Design review of the part built by this model. Coordinates are the model's own, in mm. A direction names the side the tool comes from. Give positions to 0.01 mm unless a question says otherwise; leave off trailing zeros. Write each loop counter-clockwise with the first axis right and the second up, starting at its lowest first coordinate (ties: lowest second). Pieces come first, ordered by that corner, then holes.
```python
from build123d import *
from build123d.topology import SkipClean

# Parameters (mm, degrees)
BOSS_EXTRUDE1_DEPTH          = 50
CUT_REVOLVE1_ANGLE           = 90
CUT_REVOLVE1_OTHER_WAY_ANGLE = 90
SKETCH5_R                    = 10
CUT_EXTRUDE1_DEPTH           = 524.883590244


# Read off the part's stored shape, not the designer's step: Revolve1
with BuildPart() as part:
    # Sketch1 → Boss-Extrude1 (new body)
    with BuildSketch(Plane.XY):
        Polygon((-25, -16.128), (-406.051177665, -236.128), (-421.051177665, -210.147237886), (-25, 18.513016151), (-25, 40), (25, 40), (25, -40), (-25, -40), align=None)
    extrude(amount=BOSS_EXTRUDE1_DEPTH)

    # Revolve1 outline → Revolve1 (revolve)
    with BuildSketch(Plane(origin=(-406.784806521, -234.857317547, 25), x_dir=(0.8660254037844362, 0.5000000000000042, 0), z_dir=(0, 0, -1))):
        with BuildLine():
            Line((0, 11.467257712), (0, -28.532742288))
            Line((0, -28.532742288), (40, -28.532742288))
            ThreePointArc((40, -28.532742288), (28.284271247, -0.24847104), (0, 11.467257712))
        make_face()
    revolve(axis=Axis((-406.784806521, -234.857317547, 25), (0.5000000000000042, -0.8660254037844362, 0)))

    # Sketch4 → Cut-Revolve1 (revolve, cut)
    with BuildSketch(Plane.XY.offset(25)):
        with BuildLine():
            Line((-395.706087523, -183.967237886), (-456.327865788, -218.967237886))
            ThreePointArc((-456.327865788, -218.967237886), (-408.516976655, -231.778127019), (-395.706087523, -183.967237886))
        make_face()
    revolve(axis=Axis((-395.706087523, -183.967237886, 25), (-0.8660254037844387, -0.49999999999999994, 0)), revolution_arc=CUT_REVOLVE1_ANGLE, mode=Mode.SUBTRACT)

    # Sketch4 → Cut-Revolve1 other way (revolve, cut)
    with SkipClean():  # the faces are left unmerged after this step: merging them gives an invalid solid
        with BuildSketch(Plane.XY.offset(25)):
            with BuildLine():
                Line((-395.706087523, -183.967237886), (-456.327865788, -218.967237886))
                ThreePointArc((-456.327865788, -218.967237886), (-408.516976655, -231.778127019), (-395.706087523, -183.967237886))
            make_face()
        revolve(axis=Axis((-395.706087523, -183.967237886, 25), (0.8660254037844387, 0.49999999999999994, 0)), revolution_arc=CUT_REVOLVE1_OTHER_WAY_ANGLE, mode=Mode.SUBTRACT)

    # Sketch5 → Cut-Extrude1 (cut, through all)
    with SkipClean():  # the faces are left unmerged after this step: merging them gives an invalid solid
        with BuildSketch(Plane.XY.offset(50)):
            with Locations((-111.602540378, -48.807491924)):
                Circle(SKETCH5_R)
        extrude(amount=-CUT_EXTRUDE1_DEPTH, mode=Mode.SUBTRACT)


solid = part.part
```
(1) Mouldability with a two-part tool opening along X and no side actions: class faces 1 (the face through (-118.973, -42.049, 25.35)), 2 (the face through (25, 1, 25)), 3 (the face through (-154, -85, 50)) as pulls with the +X half, pulls with the -X half, needs draft (parallel to the pull), parting line crosses it, or undercut.
Resolved:
face 1: undercut
face 2: pulls with the +X half
face 3: needs draft
(2) To check wall thickness, follow L1, parallel to Y at x = -275, z = 37.5; L2, parallel to Y at x = -66.5, z = 1; L3, parallel to X at y = -220.5, z = 42. State the ranges of each line that lie inside material, in increasing order.
Resolved:
L1: y = -160.47 to -125.82
L2: y = -40.09 to -5.45
L3: x = -402.06 to -378.98
(3) Clearance check with flat-ended pins moving along their axes: P1, Ø5, axis at x = -65, z = 53.5, coming from the -Y side; P2, Ø10, axis at x = -228, z = 33, coming from the +Y side; P3, Ø8, axis at y = -68, z = 37, coming from the +X side; P4, Ø12, axis at y = -30, z = 20.5, coming from the -X side. State where each tip first meets the part, or that it passes through.
Resolved:
P1: passes through
P2: stops at y = -95.8
P3: stops at x = -107.92
P4: stops at x = -119.42
(4) Tool access review of faces 4 (the face through (0, -40, 25)), 5 (the face through (-25, 29, 25)), 6 (the face through (0, 40, 25)): name each direction out of +Z, -Z, +X, -X, +Y, -Y from which nothing blocks a thin tool from reaching the whole face with its end or side.
Resolved:
face 4: +Z, -Z, +X, -Y
face 5: +Z, -Z, -X, +Y
face 6: +Z, -Z, +X, -X, +Y
(5) Consider section C-C, the plane y = -145. Give the boundary of the cut face in (x, z), then the cut area to 3 significant figures.
Resolved:
outline: (-308.21, 0) - (-248.21, 0) - (-248.21, 50) - (-308.21, 50) - close
area: 3,000 mm2
(6) Consider section D-D, the plane z = 13. Give the boundary of the cut face in (x, y).
Resolved:
outline: (-454.1, -229.23) arc R38.16 ccw to (-385.63, -224.34) - (-25, -16.13) - (-25, -40) - (25, -40) - (25, 40) - (-25, 40) - (-25, 18.51) - (-393.89, -194.47) arc R32.88 cw to (-448.14, -225.79) - close; hole circle Ø20 at (-111.6, -48.81)
(7) Consider section A-A, the plane z = 44. Give the boundary of the cut face in (x, y).
Resolved:
outline: (-451.53, -227.75) arc R35.2 ccw to (-390.11, -226.92) - (-25, -16.13) - (-25, -40) - (25, -40) - (25, 40) - (-25, 40) - (-25, 18.51) - (-397.08, -196.31) arc R29.39 cw to (-444.95, -223.95) - close; hole circle Ø20 at (-111.6, -48.81)
(8) Consider section B-B, the plane x = -111.5. Give the boundary of the cut face in (y, z).
Resolved:
outline: (-66.07, 0) - (-58.81, 0) - (-58.81, 50) - (-66.07, 50) - close; (-38.81, 0) - (-31.43, 0) - (-31.43, 50) - (-38.81, 50) - close
